```python
from build123d import *

# Parameters (mm, degrees)
SKETCH_1_R          = 1.5
SKETCH_1_R_2        = 25
SKETCH_1_R_3        = 1
EXTRUDE_1_DEPTH     = 2
CUT_EXTRUDE_1_DEPTH = 10
EXTRUDE_2_DEPTH     = 2
CUT_EXTRUDE_2_DEPTH = 2
CUT_EXTRUDE_3_DEPTH = 2
SKETCH_6_R          = 3
EXTRUDE_3_DEPTH     = 2


with BuildPart() as part:
    # 草图1 → 凸台-拉伸1 (new body)
    with BuildSketch(Plane(origin=(0, 0, 0), x_dir=(1, 0, 0), z_dir=(0, 1, 0))):
        with BuildLine():
            Line((-65.384333619, -19.133302588), (-28.141777015, -7.644526431))
            ThreePointArc((-28.141777015, -7.644526431), (-22.5, 0), (-28.141777015, 7.644526431))
            Line((-28.141777015, 7.644526431), (-65.384333619, 19.133302588))
            ThreePointArc((-65.384333619, 19.133302588), (-67.41435877, 22.711697239), (-63.963475544, 24.951633702))
            Line((-63.963475544, 24.951633702), (-35.956989403, 19.860837807))
            ThreePointArc((-35.956989403, 19.860837807), (-23.387681178, 22.884481961), (-17.156151846, 34.211351583))
            Line((-17.156151846, 34.211351583), (-13.884981819, 71.681117341))
            Line((-13.884981819, 71.681117341), (-12.908791343, 65.681117341))
            Line((-12.908791343, 65.681117341), (-12.384981819, 71.681117341))
            Line((-12.384981819, 71.681117341), (-11.408791343, 65.681117341))
            Line((-11.408791343, 65.681117341), (-10.884981819, 71.681117341))
            Line((-10.884981819, 71.681117341), (-10.181933712, 67.359943609))
            ThreePointArc((-10.181933712, 67.359943609), (-9.503585574, 66.157577472), (-8.20789029, 65.681117341))
            Line((-8.20789029, 65.681117341), (8.315681587, 65.681117341))
            ThreePointArc((8.315681587, 65.681117341), (9.616278401, 66.161759606), (10.291753417, 67.372669415))
            Line((10.291753417, 67.372669415), (10.964265319, 71.681117341))
            Line((10.964265319, 71.681117341), (11.488074843, 65.681117341))
            Line((11.488074843, 65.681117341), (12.424623569, 71.681117341))
            Line((12.424623569, 71.681117341), (12.948433093, 65.681117341))
            Line((12.948433093, 65.681117341), (13.884981819, 71.681117341))
            Line((13.884981819, 71.681117341), (17.156151846, 34.211351583))
            ThreePointArc((17.156151846, 34.211351583), (23.387681178, 22.884481961), (35.956989403, 19.860837807))
            Line((35.956989403, 19.860837807), (63.963475544, 24.951633702))
            ThreePointArc((63.963475544, 24.951633702), (67.41435877, 22.711697239), (65.384333619, 19.133302588))
            Line((65.384333619, 19.133302588), (28.141777015, 7.644526431))
            ThreePointArc((28.141777015, 7.644526431), (22.5, 0), (28.141777015, -7.644526431))
            Line((28.141777015, -7.644526431), (65.384333619, -19.133302588))
            ThreePointArc((65.384333619, -19.133302588), (67.41435877, -22.711697239), (63.963475544, -24.951633702))
            Line((63.963475544, -24.951633702), (58.552147091, -23.968005533))
            Line((58.552147091, -23.968005533), (55.287915388, -33.53852231))
            Line((55.287915388, -33.53852231), (55.60051339, -23.431481077))
            Line((55.60051339, -23.431481077), (52.336281687, -33.001997855))
            Line((52.336281687, -33.001997855), (52.648879688, -22.894956622))
            Line((52.648879688, -22.894956622), (49.384647985, -32.465473399))
            Line((49.384647985, -32.465473399), (49.697245987, -22.358432166))
            Line((49.697245987, -22.358432166), (31.930731882, -19.128976796))
            ThreePointArc((31.930731882, -19.128976796), (25.373883295, -20.858100658), (22.5, -27))
            Line((22.5, -27), (28, -90))
            Line((28, -90), (28, -109.5))
            ThreePointArc((28, -109.5), (24.924621202, -116.924621202), (17.5, -120))
            Line((17.5, -120), (-17.5, -120))
            ThreePointArc((-17.5, -120), (-24.924621202, -116.924621202), (-28, -109.5))
            Line((-28, -109.5), (-28, -90))
            Line((-28, -90), (-22.5, -27))
            ThreePointArc((-22.5, -27), (-25.142969185, -20.335475151), (-32.064056542, -18.464719321))
            Line((-32.064056542, -18.464719321), (-49.692991602, -22.050022904))
            Line((-49.692991602, -22.050022904), (-49.169938488, -32.148360166))
            Line((-49.169938488, -32.148360166), (-52.632809487, -22.647911521))
            Line((-52.632809487, -22.647911521), (-52.109756374, -32.746248782))
            Line((-52.109756374, -32.746248782), (-55.572627373, -23.245800138))
            Line((-55.572627373, -23.245800138), (-55.04957426, -33.344137399))
            Line((-55.04957426, -33.344137399), (-58.512445259, -23.843688755))
            Line((-58.512445259, -23.843688755), (-63.902111383, -24.939817886))
            ThreePointArc((-63.902111383, -24.939817886), (-67.406788203, -22.742012359), (-65.384333619, -19.133302588))
        make_face()
        with Locations(Location((-64.5, 22, 0), (0, 0, 270))):
            Circle(SKETCH_1_R, mode=Mode.SUBTRACT)
        with Locations(Location((64.5, 22, 0), (0, 0, 90))):
            Circle(SKETCH_1_R, mode=Mode.SUBTRACT)
        with Locations(Location((64.5, -22, 0), (0, 0, 270))):
            Circle(SKETCH_1_R, mode=Mode.SUBTRACT)
        with Locations(Location((-64.5, -22, 0), (0, 0, 90))):
            Circle(SKETCH_1_R, mode=Mode.SUBTRACT)
        with Locations(Location((0, -90, 0), (0, 0, 270))):
            Circle(SKETCH_1_R_2, mode=Mode.SUBTRACT)
        with Locations(Location((-15, -65, 0), (0, 0, 270))):
            Circle(SKETCH_1_R_3, mode=Mode.SUBTRACT)
        with Locations(Location((15, -65, 0), (0, 0, 270))):
            Circle(SKETCH_1_R_3, mode=Mode.SUBTRACT)
        with Locations(Location((-15.42, -115, 0), (0, 0, 270))):
            Circle(SKETCH_1_R_3, mode=Mode.SUBTRACT)
        with Locations(Location((17.43, -115, 0), (0, 0, 270))):
            Circle(SKETCH_1_R_3, mode=Mode.SUBTRACT)
    extrude(amount=EXTRUDE_1_DEPTH)

    # 草图2 → 切除-拉伸1 (cut)
    with BuildSketch(Plane.XZ):
        with BuildLine():
            Line((-19, 2), (-19, -18))
            ThreePointArc((-19, -18), (-19.75, -18.75), (-20.5, -18))
            Line((-20.5, -18), (-20.5, 2))
            ThreePointArc((-20.5, 2), (-19.75, 2.75), (-19, 2))
        make_face()
        with BuildLine():
            Line((20.5, 2), (20.5, -18))
            ThreePointArc((20.5, -18), (19.75, -18.75), (19, -18))
            Line((19, -18), (19, 2))
            ThreePointArc((19, 2), (19.75, 2.75), (20.5, 2))
        make_face()
        with BuildLine():
            Line((-19, 52), (-19, 32))
            ThreePointArc((-19, 32), (-19.75, 31.25), (-20.5, 32))
            Line((-20.5, 32), (-20.5, 52))
            ThreePointArc((-20.5, 52), (-19.75, 52.75), (-19, 52))
        make_face()
        with BuildLine():
            Line((20.5, 52), (20.5, 32))
            ThreePointArc((20.5, 32), (19.75, 31.25), (19, 32))
            Line((19, 32), (19, 52))
            ThreePointArc((19, 52), (19.75, 52.75), (20.5, 52))
        make_face()
        with BuildLine():
            ThreePointArc((-10, 55), (0, 45), (10, 55))
            ThreePointArc((10, 55), (0, 52.595917942), (-10, 55))
        make_face()
    extrude(amount=-CUT_EXTRUDE_1_DEPTH, mode=Mode.SUBTRACT)

    # 草图3 → 凸台-拉伸2 (add)
    with BuildSketch(Plane.XZ):
        Polygon((-1.5, 52.647113875), (0, 47.5), (1.5, 52.647113875), (1.5, 53.687015642), (2, 53.687015642), (2, 52.687015642), (3.5, 47.5), (5, 53.171632657), (5, 54.171632657), (-5, 54.171632657), (-5, 53.171632657), (-3.5, 47.5), (-2, 52.687015642), (-2, 53.687015642), (-1.5, 53.687015642), align=None)
        Polygon((-1.75, 50.5), (-0.25, 45.003125488), (-0.25, 44.003125488), (0.25, 44.003125488), (0.25, 45.003125488), (1.75, 50.5), (3.25, 45.54285984), (3.25, 43.54285984), (-3.25, 43.54285984), (-3.25, 45.54285984), align=None)
    extrude(amount=-EXTRUDE_2_DEPTH)

    # 草图4 → 切除-拉伸2 (cut)
    with BuildSketch(Plane.XZ):
        with BuildLine():
            Line((-28, 108), (-21.44761059, 108))
            ThreePointArc((-21.44761059, 108), (-26.31095871, 99.57775818), (-28, 90))
            Line((-28, 90), (-28, 108))
        make_face()
        with BuildLine():
            Line((-21.44761059, 113), (-21.44761059, 119.229664467))
            ThreePointArc((-21.44761059, 119.229664467), (-25.091953813, 116.753429347), (-27.399494937, 113))
            Line((-27.399494937, 113), (-21.44761059, 113))
        make_face()
        with BuildLine():
            Line((21.44761059, 119.229664467), (21.44761059, 113))
            Line((21.44761059, 113), (27.399494937, 113))
            ThreePointArc((27.399494937, 113), (25.091953813, 116.753429347), (21.44761059, 119.229664467))
        make_face()
        with BuildLine():
            Line((21.44761059, 108), (28, 108))
            Line((28, 108), (28, 90))
            ThreePointArc((28, 90), (26.31095871, 99.57775818), (21.44761059, 108))
        make_face()
    extrude(amount=-CUT_EXTRUDE_2_DEPTH, mode=Mode.SUBTRACT)

    # 草图5 → 切除-拉伸3 (cut)
    with BuildSketch(Plane.XZ):
        Polygon((-6, 35), (6, 35), (3, 30), (-3, 30), align=None)
        Polygon((-3, 28), (3, 28), (5, 0), (0, -6), (-5, 0), align=None)
    extrude(amount=-CUT_EXTRUDE_3_DEPTH, mode=Mode.SUBTRACT)

    # 草图6 → 凸台-拉伸3 (add)
    with BuildSketch(Plane.XZ):
        Polygon((-21.44761059, 119.229664467), (-21.44761059, 139), (-18.44761059, 142), (18.44761059, 142), (21.44761059, 139), (21.44761059, 119.229664467), align=None)
        with Locations(Location((0, 131, 0), (0, 0, 270))):
            Circle(SKETCH_6_R, mode=Mode.SUBTRACT)
    extrude(amount=-EXTRUDE_3_DEPTH)


solid = part.part
```
Geometry check sheet. Reference: the model listing, model coordinates, mm. A direction names the side the tool comes from. Round coordinates to 2 decimals unless told otherwise and drop trailing zeros. Order: outer loops, then holes, each group sorted by start corner. A loop starts at its lowest first (then second) coordinate and runs counter-clockwise, first axis right, second up. Notation, with made-up numbers: (34, -27.5) -> (54, -27.5) arc R24 ccw to (54, 3.5) -> close; hole circle Ø6 at (-32.75, -35). An arc over 180 degrees is marked (long way). Return JSON: item names as keys, results as strings. Group by question number.
Q1. Release check for a two-part mould opening along Z. For faces 1 (the flat face through (-25.29, 0.99, 58.94)), 2 (the flat face through (5, 0, 28)), 3 (the flat face through (-50.156, 0.986, -22.442)) record: released by +Z, released by -Z, zero draft, split by the parting line, or undercut.
Q2. Gauge pin test, flat ends, axial feed: pin 1 (0.6 mm diameter, centred on x = 26, y = 0.5, fed in from -Z); pin 2 (1 mm diameter, centred on x = -26, y = 0.5, fed in from -Z); pin 3 (1 mm diameter, centred on x = 26, y = 0.5, fed in from +Z). Record the tip position at first contact, or that the pin passes through.
Q3. Section check A-A, the plane z = 95. Record the boundary of the cut face in (x, y).
Q4. Tool access check on faces 4 (the flat face through (46.502, 0.986, 13.308)), 5 (the cylindrical face through (25.45, 0.986, 20.796)), 6 (the flat face through (49.76, 0.99, -22.37)), 7 (the flat face through (-47.02, 0.99, 13.47)). Record the directions out of +Z, -Z, +X, -X, +Y, -Y that give a thin tool (end or side, any length) a straight path to the whole face; none if there is none.
Q5. Material ranges on probe 1 along X at (y, z) = (0.9, 131); probe 2 along Z at (x, y) = (-64.5, 0.5); probe 3 along X at (y, z) = (1, 90), recorded low to high. Write a range as from..to.
Q6. Section check D-D, the plane z = -53.5. Record the boundary of the cut face in (x, y).
Q7. Section check B-B, the plane y = 0.8. Count the separate pieces of the cut face and the enclosed holes in it, plus the area to 3 significant figures.
Q8. Section check C-C, the plane z = 122.5. Record the boundary of the cut face in (x, y).
Numbers:
{
 "1": {"face 1": "undercut", "face 2": "zero draft", "face 3": "released by -Z"},
 "2": {"pin 1": "z = -21.41", "pin 2": "z = -21.52", "pin 3": "z = 113"},
 "3": {"outline": "(-27.55, 0) -> (-24.49, 0) -> (-24.49, 2) -> (-27.55, 2) -> close; (24.49, 0) -> (27.55, 0) -> (27.55, 2) -> (24.49, 2) -> close"},
 "4": {"face 4": "+X, +Y, -Y", "face 5": "+Y, -Y", "face 6": "-Z, +Y, -Y", "face 7": "-X, +Y, -Y"},
 "5": {"probe 1": "-21.45..-3, 3..21.45", "probe 2": "-25..-23.5, -20.5..-18.86, 18.86..20.5, 23.5..25", "probe 3": "-28..-25, 25..28"},
 "6": {"outline": "(-15.47, 0) -> (15.47, 0) -> (15.47, 2) -> (-15.47, 2) -> close"},
 "7": {"separate pieces": "1", "enclosed holes": "17", "area": "8,520 mm^2"},
 "8": {"outline": "(-21.45, 0) -> (21.45, 0) -> (21.45, 2) -> (-21.45, 2) -> close"}
}
